CAD build for the part. Positions are in the model's coordinates, mm. A direction names the side the tool comes from. Give positions to 0.01 mm unless a question says otherwise; leave off trailing zeros. Write each loop counter-clockwise with the first axis right and the second up, starting at its lowest first coordinate (ties: lowest second). Pieces come first, ordered by that corner, then holes. Notation, with made-up numbers: M 22.25,-18.75 L 75.25,-18.75 A23 cw 75.25,-6.75 Z; hole C 25.25,86 d10. An arc over 180 degrees is marked long. One line per question, with ' | ' between items. Start each with the question number.
1. Wall check: L1, parallel to Y at x = 39, z = 3. Give the ranges that are in metal, low to high.
2. Cut at A-A, the plane y = 10.5. Count the separate pieces of the cut face and the enclosed holes in it, then the cut area to 3 significant figures.
3. Flat gauge pin, fed straight in: pin 1 (1.5 mm diameter, centred on x = -37, z = 1.5, fed in from +Y). Where does the tip first touch, or does it go through?
4. Pull direction X, two halves, no side cores. Call faces 3 (the face through (20.2, 11, 2)), 4 (the face through (60.8, 8, 2)), 5 (the face through (58, 15, 2)): released by +X, released by -X, zero draft, split by the parting line, or undercut.
5. Cut at C-C, the plane x = 7.5. Write the cut outline in (y, z).
6. Which spindle directions (+Z, -Z, +X, -X, +Y, -Y) get a long thin tool onto all of the face, cutting with end or side? Do faces 1 (the face through (53, 7.5, 2)), 2 (the face through (0, 15, 2)). Say none if no direction does.
Autodesk Inventor part; units mm, degrees
ref_plane "YZ Plane" through (0, 0, 0) normal (1, 0, 0) x (0, 1, 0)
ref_plane "XZ Plane" through (0, 0, 0) normal (0, 1, 0) x (-1, 0, 0)
ref_plane "XY Plane" through (0, 0, 0) normal (0, 0, 1) x (1, 0, 0)
sketch "Sketch1" plane through (0, 0, 0) normal (0, 0, 1) x (1, 0, 0)
  line L0 (0, 0) -> (0, 15)
  line L1 (0, 15) -> (5, 15)
  line L2 (5, 15) -> (5, 7.5)
  line L3 (5, 7.5) -> (10.2, 7.5)
  line L4 (10.2, 7.5) -> (10.2, 15)
  line L5 (10.2, 15) -> (15.2, 15)
  line L6 (15.2, 15) -> (15.2, 0)
  line L7 (15.2, 0) -> (0, 0)
  dimension "d0" = 15
  dimension "d1" = 5.2
  dimension "d2" = 5
  dimension "d3" = 5
  dimension "d4" = 7.5
extrude "Extrusion1" add sketch "Sketch1" along normal blind 5
mirror "Mirror1" about plane through (15.2, 0, 0) normal (1, 0, 0) of "Extrusion1"
mirror "Mirror2" about plane through (30.4, 15, 0) normal (1, 0, 0) of "Extrusion1", "Mirror1"
mirror "Mirror4" about plane through (0, 15, 0) normal (-1, 0, 0) of "Extrusion1"
mirror "Mirror5" about plane through (-15.2, 0, 0) normal (-1, 0, 0) of "Extrusion1", "Mirror4"
ref_plane "Work Plane3" through (45.6, 7.5, 0) normal (1, 0, 0) x (0, 0, -1)
properties part number "brace"
Here are the results:
1) L1: 0 to 7.5
2) separate pieces: 8 | enclosed holes: 0 | area: 350 mm^2
3) pin 1: y = 7.5
4) face 3: undercut | face 4: released by +X | face 5: zero draft
5) outline: M 0,0 L 7.5,0 L 7.5,5 L 0,5 Z
6) face 1: +Z, -Z, +Y | face 2: +Z, -Z, +X, -X, +Y
